Part model, mm, in its own coordinate system. Face numbers are marked on the shaded views. A direction names the side the tool comes from. Round coordinates to 2 decimals unless told otherwise and drop trailing zeros. Write each loop counter-clockwise with the first axis right and the second up, starting at its lowest first coordinate (ties: lowest second). Pieces come first, ordered by that corner, then holes.
```python
from build123d import *

# Parameters (mm, degrees)
SKETCH1_W           = 175
SKETCH1_H           = 90
BOSS_EXTRUDE1_DEPTH = 90
CUT_EXTRUDE1_DEPTH  = 90
SKETCH3_W           = 40
SKETCH3_H           = 30
CUT_EXTRUDE2_DEPTH  = 90
SKETCH4_W           = 25
SKETCH4_H           = 5
CUT_EXTRUDE3_DEPTH  = 90
CUT_EXTRUDE4_DEPTH  = 70
CUT_EXTRUDE5_DEPTH  = 308
CUT_EXTRUDE6_DEPTH  = 30
CUT_EXTRUDE7_DEPTH  = 25
CUT_EXTRUDE8_DEPTH  = 15
SKETCH10_W          = 45
SKETCH10_H          = 90
CUT_EXTRUDE9_DEPTH  = 154
BOSS_EXTRUDE2_DEPTH = 25
CUT_EXTRUDE10_DEPTH = 15
SKETCH13_W          = 30.156865167
SKETCH13_H          = 5
BOSS_EXTRUDE3_DEPTH = 25


with BuildPart() as part:
    # Sketch1 → Boss-Extrude1 (new body)
    with BuildSketch(Plane.XY):
        with Locations((87.5, 45)):
            Rectangle(SKETCH1_W, SKETCH1_H)
    extrude(amount=BOSS_EXTRUDE1_DEPTH)

    # Sketch2 → Cut-Extrude1 (cut)
    with BuildSketch(Plane.XY.offset(90)):
        with BuildLine():
            Line((45, 90), (0, 90))
            Line((0, 90), (0, 45))
            ThreePointArc((0, 45), (13.180194847, 76.819805153), (45, 90))
        make_face()
        with BuildLine():
            ThreePointArc((45, 0), (13.180194847, 13.180194847), (0, 45))
            Line((0, 45), (0, 0))
            Line((0, 0), (45, 0))
        make_face()
    extrude(amount=-CUT_EXTRUDE1_DEPTH, mode=Mode.SUBTRACT)

    # Sketch3 → Cut-Extrude2 (cut)
    with BuildSketch(Plane.XY.offset(90)):
        with Locations((155, 75)):
            Rectangle(SKETCH3_W, SKETCH3_H)
        with Locations((155, 15)):
            Rectangle(SKETCH3_W, SKETCH3_H)
    extrude(amount=-CUT_EXTRUDE2_DEPTH, mode=Mode.SUBTRACT)

    # Sketch4 → Cut-Extrude3 (cut)
    with BuildSketch(Plane.XY.offset(90)):
        with Locations((162.5, 57.5)):
            Rectangle(SKETCH4_W, SKETCH4_H)
        with Locations((162.5, 32.5)):
            Rectangle(SKETCH4_W, SKETCH4_H)
    extrude(amount=-CUT_EXTRUDE3_DEPTH, mode=Mode.SUBTRACT)

    # Sketch5 → Cut-Extrude4 (cut)
    with BuildSketch(Plane.XY.offset(90)):
        with BuildLine():
            ThreePointArc((16.715728753, 10), (31.00858661, 45), (16.715728753, 80))
            ThreePointArc((16.715728753, 80), (0, 45), (16.715728753, 10))
        make_face()
    extrude(amount=-CUT_EXTRUDE4_DEPTH, mode=Mode.SUBTRACT)

    # Sketch6 → Cut-Extrude5 (cut)
    with BuildSketch(Plane(origin=(0, 0, 0), x_dir=(0, 0, -1), z_dir=(1, 0, 0))):
        with BuildLine():
            Line((-82.336131476, 60.742295265), (-45, 90))
            Line((-45, 90), (-90, 90))
            Line((-90, 90), (-90, 45))
            ThreePointArc((-90, 45), (-87.982249992, 53.75435236), (-82.336131476, 60.742295265))
        make_face()
        with BuildLine():
            ThreePointArc((-82.336131476, 29.257704735), (-87.982249992, 36.24564764), (-90, 45))
            Line((-90, 45), (-90, 0))
            Line((-90, 0), (-45, 0))
            Line((-45, 0), (-82.336131476, 29.257704735))
        make_face()
    extrude(amount=CUT_EXTRUDE5_DEPTH, mode=Mode.SUBTRACT)

    # Sketch7 → Cut-Extrude6 (cut)
    with BuildSketch(Plane(origin=(0, 0, 0), x_dir=(-1, 0, 0), z_dir=(0, 0, -1))):
        with BuildLine():
            Line((-135, 75), (-45, 75))
            ThreePointArc((-45, 75), (-15, 45), (-45, 15))
            Line((-45, 15), (-135, 15))
            Line((-135, 15), (-135, 75))
        make_face()
    extrude(amount=-CUT_EXTRUDE6_DEPTH, mode=Mode.SUBTRACT)

    # Sketch8 → Cut-Extrude7 (cut)
    with BuildSketch(Plane(origin=(175, 0, 0), x_dir=(0, 0, -1), z_dir=(1, 0, 0))):
        with BuildLine():
            Line((-70, 55), (-87.320508076, 55))
            ThreePointArc((-87.320508076, 55), (-90, 45), (-87.320508076, 35))
            Line((-87.320508076, 35), (-70, 35))
            ThreePointArc((-70, 35), (-80, 45), (-70, 55))
        make_face()
        with BuildLine():
            Line((0, 55), (-70, 55))
            ThreePointArc((-70, 55), (-62.928932188, 52.071067812), (-60, 45))
            ThreePointArc((-60, 45), (-62.928932188, 37.928932188), (-70, 35))
            Line((-70, 35), (0, 35))
            Line((0, 35), (0, 55))
        make_face()
    extrude(amount=-CUT_EXTRUDE7_DEPTH, mode=Mode.SUBTRACT)

    # Sketch9 → Cut-Extrude8 (cut)
    with BuildSketch(Plane(origin=(150, 0, 0), x_dir=(0, 0, -1), z_dir=(1, 0, 0))):
        with BuildLine():
            Line((-70, 60), (-83.228756555, 60))
            ThreePointArc((-83.228756555, 60), (-90, 45), (-83.228756555, 30))
            Line((-83.228756555, 30), (-70, 30))
            ThreePointArc((-70, 30), (-85, 45), (-70, 60))
        make_face()
        with BuildLine():
            Line((0, 60), (-70, 60))
            ThreePointArc((-70, 60), (-59.393398282, 55.606601718), (-55, 45))
            ThreePointArc((-55, 45), (-59.393398282, 34.393398282), (-70, 30))
            Line((-70, 30), (0, 30))
            Line((0, 30), (0, 60))
        make_face()
    extrude(amount=-CUT_EXTRUDE8_DEPTH, mode=Mode.SUBTRACT)

    # Sketch10 → Cut-Extrude9 (cut)
    with BuildSketch(Plane(origin=(115, 0, 0), x_dir=(0, 0, -1), z_dir=(1, 0, 0))):
        with Locations((-67.5, 45)):
            Rectangle(SKETCH10_W, SKETCH10_H)
    extrude(amount=-CUT_EXTRUDE9_DEPTH, mode=Mode.SUBTRACT)

    # Sketch11 → Boss-Extrude2 (add)
    with BuildSketch(Plane.XY.offset(45)):
        with BuildLine():
            Line((65, 55), (65, 65))
            ThreePointArc((65, 65), (85, 45), (65, 25))
            Line((65, 25), (65, 35))
            ThreePointArc((65, 35), (75, 45), (65, 55))
        make_face()
    extrude(amount=BOSS_EXTRUDE2_DEPTH)

    # Sketch12 → Cut-Extrude10 (cut)
    with BuildSketch(Plane.XY.offset(45)):
        with BuildLine():
            Line((65, 35), (45, 35))
            ThreePointArc((45, 35), (35, 45), (45, 55))
            Line((45, 55), (65, 55))
            ThreePointArc((65, 55), (75, 45), (65, 35))
        make_face()
    extrude(amount=-CUT_EXTRUDE10_DEPTH, mode=Mode.SUBTRACT)

    # Sketch13 → Boss-Extrude3 (add)
    with BuildSketch(Plane.XY.offset(45)):
        with Locations((99.921567417, 45)):
            Rectangle(SKETCH13_W, SKETCH13_H)
    extrude(amount=BOSS_EXTRUDE3_DEPTH)


solid = part.part
```
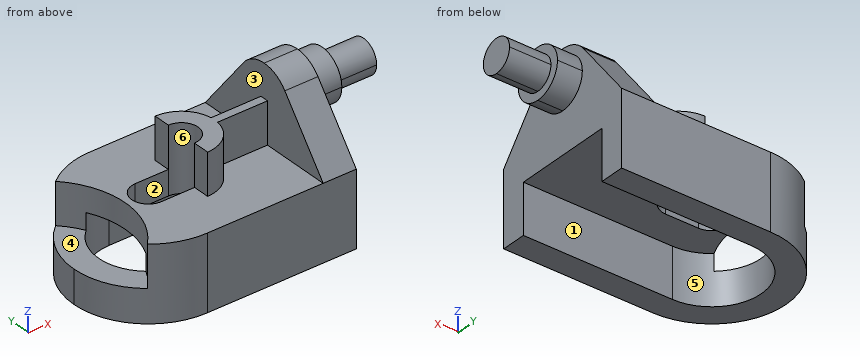
Q1. Cut at D-D on x = 94. Write the cut outline in (y, z).
Values follow:
outline: (0, 0) - (15, 0) - (15, 30) - (75, 30) - (75, 0) - (90, 0) - (90, 45) - (47.5, 45) - (47.5, 70) - (42.5, 70) - (42.5, 45) - (0, 45) - close
Q2. Which spindle directions (+Z, -Z, +X, -X, +Y, -Y) get a long thin tool onto all of the face, cutting with end or side? Do the marked faces 1, 2 and 3. Say none if no direction does.
Values follow:
face 1: -Z, +X
face 2: +Z, -Z
face 3: +Z
Q3. Drop flat-ended pins along their axis: pin 1 (5 mm diameter, centred on y = 31, z = 54.5, fed in from -X); pin 2 (6 mm diameter, centred on x = 55.5, y = 55, fed in from -Z); pin 3 (5 mm diameter, centred on y = 55, z = 45, fed in from +X). Give the stop position or say it passes through.
Values follow:
pin 1: stops at x = 65
pin 2: stops at z = 30
pin 3: stops at x = 135
Q4. Mould opens along X. For the marked faces 4, 5 and 6 say: +X half, -X half, draft (parallel to the pull), parting line (faces both ways), or undercut.
Values follow:
face 4: draft
face 5: +X half
face 6: undercut
Q5. Cut at B-B on z = 17. Write the cut outline in (x, y).
Values follow:
outline: (45, 0) - (135, 0) - (135, 15) - (45, 15) arc R30 cw to (45, 75) - (135, 75) - (135, 90) - (45, 90) arc R45 ccw to start
Q6. Wall check: L1, parallel to Z at x = 48, y = 20; L2, parallel to X at y = 50, z = 79; L3, parallel to X at y = 53, z = 70.5. Give the ranges that are in metal, low to high.
Values follow:
L1: z = 30 to 45
L2: x = 115 to 150
L3: x = 115 to 175
Q7. Cut at C-C on y = 53. Write the cut outline in (x, z), plus the area to 3 significant figures.
Values follow:
outline: (0.72, 0) - (16.09, 0) - (16.09, 20) - (0.72, 20) - close; (30.36, 30) - (39, 30) - (39, 45) - (30.36, 45) - close; (71, 30) - (135, 30) - (135, 57.31) - (150, 57.31) - (150, 64) - (175, 64) - (175, 76) - (150, 76) - (150, 82.69) - (135, 82.69) - (135, 88.33) - (115, 88.33) - (115, 45) - (83.33, 45) - (83.33, 70) - (71, 70) - close
area: 3,250 mm2
Q8. Cut at A-A on x = 48. Write the cut outline in (y, z).
Values follow:
outline: (0, 0) - (15, 0) - (15, 30) - (35, 30) - (35, 45) - (0, 45) - close; (55, 30) - (75, 30) - (75, 0) - (90, 0) - (90, 45) - (55, 45) - close
